```python
from build123d import *

# Parameters (mm, degrees)
F0_R     = 152.4
F1_DEPTH = 635
F2_W     = 560.6032549905
F2_H     = 203.2
F2_W_2   = 2.5960083008
F3_DEPTH = 317.5
F4_R     = 381


with BuildPart() as f1:
    # F0 (on Front) → F1 (new body)
    with BuildSketch(Plane.XZ):
        with BuildLine():
            ThreePointArc((243.9590334462, -203.2), (298.5491945385, -108.0491945385), (317.5, 0))
            ThreePointArc((317.5, 0), (298.5491945385, 108.0491945385), (243.9590334462, 203.2))
            ThreePointArc((243.9590334462, 203.2), (-317.5, 0), (243.9590334462, -203.2))
        make_face()
        Circle(F0_R, mode=Mode.SUBTRACT)
        with BuildLine():
            ThreePointArc((243.9590334462, 203.2), (298.5491945385, 108.0491945385), (317.5, 0))
            ThreePointArc((317.5, 0), (298.5491945385, -108.0491945385), (243.9590334462, -203.2))
            Line((243.9590334462, -203.2), (2006.6, -203.2))
            ThreePointArc((2006.6, -203.2), (1905, 0), (2006.6, 203.2))
            Line((2006.6, 203.2), (243.9590334462, 203.2))
        make_face()
        with BuildLine():
            ThreePointArc((2413, 0), (2272.592253257, 227.184506514), (2006.6, 203.2))
            ThreePointArc((2006.6, 203.2), (1905, 0), (2006.6, -203.2))
            ThreePointArc((2006.6, -203.2), (2272.592253257, -227.184506514), (2413, 0))
        make_face()
        with Locations((2159, 0)):
            Circle(F0_R, mode=Mode.SUBTRACT)
    extrude(amount=F1_DEPTH)

    # F2 (on Top) → F3 (intersect, symmetric)
    with BuildSketch(Plane.XY):
        with Locations((-36.342594049, -101.6)):
            Rectangle(F2_W, F2_H)
        Polygon((508, 0), (243.9590334462, 0), (243.9590334462, -203.2), (490.2223035715, -203.2), (1786.6773275361, -431.8), (2413, -431.8), (2413, -228.6), (1804.4550239646, -228.6), align=None)
        with Locations((2414.2980041504, -330.2)):
            Rectangle(F2_W_2, F2_H)
    extrude(amount=F3_DEPTH, both=True, mode=Mode.INTERSECT)

    # F4
    f4_edges = [f1.edges().sort_by_distance(p)[0] for p in [
        (508, 0, 0),
        (1804.455024, -228.6, 0),
        (490.222304, -203.2, 0),
        (1786.677328, -431.8, 0),
        (243.959033, -101.6, 203.2),
        (2006.6, -330.2, 203.2),
        (2006.6, -330.2, -203.2),
        (243.959033, -101.6, -203.2),
    ]]
    fillet(f4_edges, radius=F4_R)


solid = f1.part
```
Geometry: final body of the model. Coordinates: model frame, mm. A direction names the side the tool comes from. Coordinates: 2 decimals unless noted, no trailing zeros. Write each loop counter-clockwise with the first axis right and the second up, starting at its lowest first coordinate (ties: lowest second). Pieces come first, ordered by that corner, then holes. Notation, with made-up numbers: M 1.5,-11 L 39.5,-11 A26 cw 39.5,4 Z; hole C 71.25,78 d6. An arc over 180 degrees is marked long. Answer as CSV lines item,"result". Start each with the question number.
Q1. Cut plane C-C on y = -389. Return the cut outline in (x, z).
Q2. Cut plane A-A on x = 0. Return the cut outline in (y, z).
Q3. Cut plane B-B on z = 0. Return the cut outline in (x, y), then the cut area to 3 significant figures.
Q4. Mould query, pull axis X, two halves, no side actions, for faces 5 (the flat face through (161, 0, 4)), 6 (the cylindrical face through (2412.903, -328.778, -7.017)), 7 (the cylindrical face through (1985.279, -331.622, -210.684)), 8 (the cylindrical face through (-120.94, -100.18, -92.73)). Classes: released by +X, released by -X, zero draft, split by the parting line, or undercut.
Q5. Cut plane D-D on x = 2159. Return the cut outline in (y, z).
Q6. Reachability of faces 1 (the flat face through (2002, -228.6, 4)), 2 (the flat face through (151, -203.2, -66)), 3 (the flat face through (1981, -431.8, 4)), 4 (the flat face through (1136, -213, -203.2)) from +Z, -Z, +X, -X, +Y, -Y: full face, straight path, thin tool, end or side. Return the list, or none.
Q7. Line query: line 1 (Z direction, x = 0, y = -141); line 2 (Z direction, x = 2159, y = -322); line 3 (Z direction, x = 827, y = -108.5). Output: solid intervals per line, ascending. Write a range as from..to.
Q8. Pin query (flat end, axial travel): P1, Ø10, axis at x = 725.5, z = -62, coming from the -Y side; P2, Ø1, axis at x = 236.5, z = 158, coming from the -Y side; P3, Ø12, axis at x = 1751, z = -2, coming from the +Y side. Return the tip coordinate at first contact, or that it passes through.
Findings below:
1,outline,"M 1543.95,-203.2 L 1910.13,-203.2 A381 cw 2059.45,-233.68 A254 ccw long 2059.45,233.68 A381 cw 1910.13,203.2 L 1543.95,203.2 Z; hole C 2159,0 d304.8"
2,outline,"M -203.2,-317.5 L 0,-317.5 L 0,-152.4 L -203.2,-152.4 Z; M -203.2,152.4 L 0,152.4 L 0,317.5 L -203.2,317.5 Z"
3,outline,"M -316.64,-203.2 L -152.4,-203.2 L -152.4,0 L -316.64,0 Z; M 152.4,-203.2 L 456.89,-203.2 A381 cw 523.05,-208.99 L 1753.85,-426.01 A381 ccw 1820.01,-431.8 L 2006.6,-431.8 L 2006.6,-228.6 L 1837.79,-228.6 A381 cw 1771.63,-222.81 L 540.83,-5.79 A381 ccw 474.67,0 L 152.4,0 Z; M 2311.4,-431.8 L 2413,-431.8 L 2413,-228.6 L 2311.4,-228.6 Z"
3,area,"435,000 mm2"
4,face 5,"zero draft"
4,face 6,"split by the parting line"
4,face 7,"released by -X"
4,face 8,"undercut"
5,outline,"M -431.8,-254 L -228.6,-254 L -228.6,-152.4 L -431.8,-152.4 Z; M -431.8,152.4 L -228.6,152.4 L -228.6,254 L -431.8,254 Z"
6,face 1,"+Z, -Z, +X, +Y"
6,face 2,"+Z, -Z, -X, -Y"
6,face 3,"+Z, -Z, +X, -X, -Y"
6,face 4,"-Z, +Y, -Y"
7,line 1,"z = -317.5..-152.4, 152.4..317.5"
7,line 2,"z = -254..-152.4, 152.4..254"
7,line 3,"z = -203.2..203.2"
8,P1,"stops at y = -245.57"
8,P2,"stops at y = -203.2"
8,P3,"stops at y = -218.12"
